CAD build for the part. Positions are in the model's coordinates, mm. Face numbers are marked on the shaded views. Coordinates: 2 decimals unless noted, no trailing zeros. Order: outer loops, then holes, each group sorted by start corner. A loop starts at its lowest first (then second) coordinate and runs counter-clockwise, first axis right, second up. Notation, with made-up numbers: M 56,-7.75 L 111,-7.75 A21 ccw 111,16.25 Z; hole C 59.5,50.5 d5. An arc over 180 degrees is marked long. Write item = value, one per line.
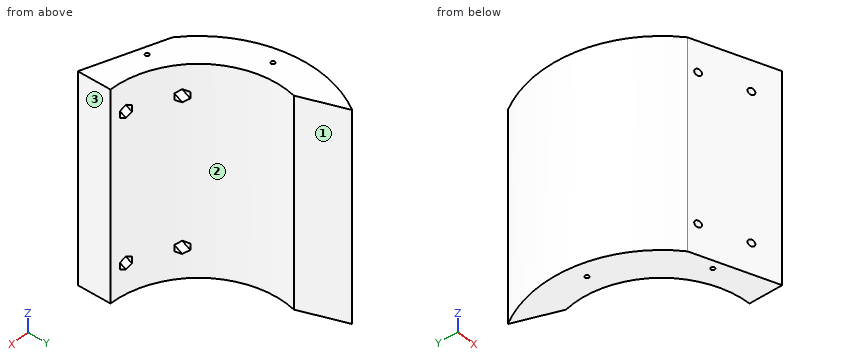
from build123d import *

# Parameters (mm, degrees)
BOSS_EXTRUDE1_DEPTH = 102.8
CUT_EXTRUDE1_DEPTH  = 103.8
CUT_EXTRUDE2_DEPTH  = 103.8
CUT_EXTRUDE3_REACH  = 87.538
SKETCH5_R           = 1.65
CUT_EXTRUDE4_START  = -5
CUT_EXTRUDE4_DEPTH  = 81.538495947
SKETCH7_R           = 0.95
CUT_EXTRUDE5_DEPTH  = 103.8


with BuildPart() as part:
    # Sketch1 → Boss-Extrude1 (new body)
    with BuildSketch(Plane.XY):
        with BuildLine():
            Line((0, 59), (0, 43))
            ThreePointArc((0, 43), (-43, 0), (0, -43))
            Line((0, -43), (0, -59))
            ThreePointArc((0, -59), (-59, 0), (0, 59))
        make_face()
    extrude(amount=BOSS_EXTRUDE1_DEPTH)

    # Sketch3 → Cut-Extrude1 (cut, through all)
    with BuildSketch(Plane.XY.offset(102.8)):
        Polygon((0, 0), (0, 90), (-70.757321084, 90), (-38, 0), align=None)
    extrude(amount=-CUT_EXTRUDE1_DEPTH, mode=Mode.SUBTRACT)

    # Sketch4 → Cut-Extrude2 (cut, through all)
    with BuildSketch(Plane.XY.offset(102.8)):
        Polygon((0, -59), (-37.631699217, -45.440677966), (-42.517346633, -59), align=None)
    extrude(amount=-CUT_EXTRUDE2_DEPTH, mode=Mode.SUBTRACT)

    # Sketch5 → Cut-Extrude3 (cut, up to next)
    with BuildSketch(Plane(origin=(-18.815849609, -52.220338983, 0), x_dir=(0.94079248, -0.338983051, 0), z_dir=(-0.338983051, -0.94079248, 0)), mode=Mode.PRIVATE) as cut_extrude3_sk1:
        with Locations((7, 15)):
            Circle(SKETCH5_R)
    cut_extrude3_tool1 = extrude(cut_extrude3_sk1.sketch, amount=-CUT_EXTRUDE3_REACH, mode=Mode.PRIVATE) & part.part
    add(cut_extrude3_tool1.solids().sort_by_distance((-12.230302, -54.59322, 15))[0], mode=Mode.SUBTRACT)
    # Sketch5 → Cut-Extrude3 (cut, up to next)
    with BuildSketch(Plane(origin=(-18.815849609, -52.220338983, 0), x_dir=(0.94079248, -0.338983051, 0), z_dir=(-0.338983051, -0.94079248, 0)), mode=Mode.PRIVATE) as cut_extrude3_sk2:
        with Locations((-15.5, 15)):
            Circle(SKETCH5_R)
    cut_extrude3_tool2 = extrude(cut_extrude3_sk2.sketch, amount=-CUT_EXTRUDE3_REACH, mode=Mode.PRIVATE) & part.part
    add(cut_extrude3_tool2.solids().sort_by_distance((-33.398133, -46.966102, 15))[0], mode=Mode.SUBTRACT)
    # Sketch5 → Cut-Extrude3 (cut, up to next)
    with BuildSketch(Plane(origin=(-18.815849609, -52.220338983, 0), x_dir=(0.94079248, -0.338983051, 0), z_dir=(-0.338983051, -0.94079248, 0)), mode=Mode.PRIVATE) as cut_extrude3_sk3:
        with Locations((-15.5, 87.8)):
            Circle(SKETCH5_R)
    cut_extrude3_tool3 = extrude(cut_extrude3_sk3.sketch, amount=-CUT_EXTRUDE3_REACH, mode=Mode.PRIVATE) & part.part
    add(cut_extrude3_tool3.solids().sort_by_distance((-33.398133, -46.966102, 87.8))[0], mode=Mode.SUBTRACT)
    # Sketch5 → Cut-Extrude3 (cut, up to next)
    with BuildSketch(Plane(origin=(-18.815849609, -52.220338983, 0), x_dir=(0.94079248, -0.338983051, 0), z_dir=(-0.338983051, -0.94079248, 0)), mode=Mode.PRIVATE) as cut_extrude3_sk4:
        with Locations((7, 87.8)):
            Circle(SKETCH5_R)
    cut_extrude3_tool4 = extrude(cut_extrude3_sk4.sketch, amount=-CUT_EXTRUDE3_REACH, mode=Mode.PRIVATE) & part.part
    add(cut_extrude3_tool4.solids().sort_by_distance((-12.230302, -54.59322, 87.8))[0], mode=Mode.SUBTRACT)

    # Sketch6 → Cut-Extrude4 (cut, through all)
    with BuildSketch(Plane(origin=(-18.815849609, -52.220338983, 0), x_dir=(0.94079248, -0.338983051, 0), z_dir=(-0.338983051, -0.94079248, 0)).offset(CUT_EXTRUDE4_START)):
        Polygon((7, 11.824573519), (9.75, 13.41228676), (9.75, 16.58771324), (7, 18.175426481), (4.25, 16.58771324), (4.25, 13.41228676), align=None)
        Polygon((-15.5, 11.824573519), (-12.75, 13.41228676), (-12.75, 16.58771324), (-15.5, 18.175426481), (-18.25, 16.58771324), (-18.25, 13.41228676), align=None)
        Polygon((-18.25, 89.38771324), (-15.5, 90.975426481), (-12.75, 89.38771324), (-12.75, 86.21228676), (-15.5, 84.624573519), (-18.25, 86.21228676), align=None)
        Polygon((4.25, 89.38771324), (7, 90.975426481), (9.75, 89.38771324), (9.75, 86.21228676), (7, 84.624573519), (4.25, 86.21228676), align=None)
    extrude(amount=-CUT_EXTRUDE4_DEPTH, mode=Mode.SUBTRACT)

    # Sketch7 → Cut-Extrude5 (cut, through all)
    with BuildSketch(Plane(origin=(0, 0, 0), x_dir=(-1, 0, 0), z_dir=(0, 0, -1))):
        with Locations((24, -46)):
            Circle(SKETCH7_R)
        with Locations((51, -8)):
            Circle(SKETCH7_R)
    extrude(amount=-CUT_EXTRUDE5_DEPTH, mode=Mode.SUBTRACT)


solid = part.part
(1) Slice it at A-A, the plane z = 37.5. Write the cut outline in (x, y), then the cut area to 3 significant figures.
Evaluation:
outline = M -49.62,31.92 A59 ccw -37.63,-45.44 L 0,-59 L 0,-43 A43 cw -41.75,10.3 Z; hole C -51,-8 d1.9; hole C -24,-46 d1.9
area = 1,540 mm²
(2) Wall check: line 1 (Y direction, x = -51, z = 47.5); line 2 (Y direction, x = -24, z = 58); line 3 (Y direction, x = -37, z = 28.5). Give the ranges that are in metal, low to high. Write a range as from..to.
Evaluation:
line_1 = -29.66..-8.95, -7.05..29.66
line_2 = -50.35..-46.95, -45.05..-35.68
line_3 = -45.67..-21.91
(3) Pin check, flat tips, straight feed: pin 1 Ø8 at (y, z) = (0.5, 53.5) entering from +X; pin 2 Ø12 at (x, z) = (-40, 86) entering from -Y; pin 3 Ø12 at (x, z) = (-10, 28) entering from +Y. Stop position of each tip, or through.
Evaluation:
pin_1 = -42.76
pin_2 = -46.75
pin_3 = -39.91
(4) Pull direction Y, two halves, no side cores. Call the marked faces 1, 2 and 3: +Y half, -Y half, draft (parallel to the pull), parting line (faces both ways), or undercut.
Evaluation:
face_1 = +Y half
face_2 = undercut
face_3 = draft
(5) Slice it at B-B, the plane y = -13. Write the cut outline in (x, z), then the cut area to 3 significant figures.
Evaluation:
outline = M -57.55,0 L -40.99,0 L -40.99,102.8 L -57.55,102.8 Z
area = 1,700 mm²
